Read the model definition and answer for the solid it produces. Units are mm, in the model's axes. Face numbers are marked on the shaded views. A direction names the side the tool comes from. Round coordinates to 2 decimals unless told otherwise and drop trailing zeros. Loops run counter-clockwise (first coordinate to the right, second up) from the corner with the lowest first, then second, coordinate; pieces in that order, holes last. Notation, with made-up numbers: M 47.25,-1 L 80.25,-1 A11 ccw 80.25,7 Z; hole C 60,64.25 d1. An arc over 180 degrees is marked long. Write each question's results on one line, items separated by ' | '.
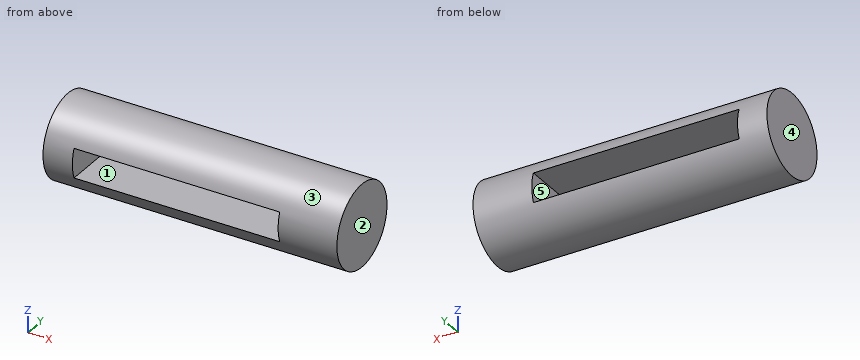
```python
from build123d import *

# Parameters (mm, degrees)
SKETCH1_R           = 7
BOSS_EXTRUDE1_DEPTH = 50
SKETCH2_W           = 35
SKETCH2_H           = 14
CUT_EXTRUDE1_DEPTH  = 2.5


with BuildPart() as part:
    # Sketch1 → Boss-Extrude1 (new body)
    with BuildSketch(Plane(origin=(0, 0, 0), x_dir=(0, 0, -1), z_dir=(1, 0, 0))):
        Circle(SKETCH1_R)
    extrude(amount=BOSS_EXTRUDE1_DEPTH)

    # Sketch2 → Cut-Extrude1 (cut, symmetric)
    with BuildSketch(Plane.XY):
        with Locations((22.5, 0)):
            Rectangle(SKETCH2_W, SKETCH2_H)
    extrude(amount=CUT_EXTRUDE1_DEPTH, both=True, mode=Mode.SUBTRACT)


solid = part.part
```
1. Find section B-B, the plane y = 2.5. Give the vertices of the cut face in (x, z), then the cut area to 3 significant figures.
Completed:
outline: M 0,-6.54 L 50,-6.54 L 50,6.54 L 0,6.54 Z; hole M 5,-2.5 L 40,-2.5 L 40,2.5 L 5,2.5 Z | area: 479 mm2
2. Given P1, Ø8, axis at x = 7, y = 4.5, coming from the +Z side; P2, Ø5, axis at x = 6.5, z = 3.5, coming from the -Y side; P3, Ø1, axis at x = 43.5, y = 5, coming from the +Z side, each flat-ended and moving along its own axis, determine where each tip first touches the part or whether it passes through.
Completed:
P1: stops at z = 6.98 | P2: stops at y = -6.84 | P3: stops at z = 5.36
3. Find section A-A, the plane z = 0. Give the vertices of the cut face in (x, y), then the cut area to 3 significant figures.
Completed:
outline: M 0,-7 L 5,-7 L 5,7 L 0,7 Z; M 40,-7 L 50,-7 L 50,7 L 40,7 Z | area: 210 mm2
4. Find section C-C, the plane x = 33. Give the vertices of the cut face in (y, z).
Completed:
outline: M -6.54,-2.5 A7 ccw 6.54,-2.5 Z; M -6.54,2.5 L 6.54,2.5 A7 ccw Z
5. Determine the mould class of the marked faces 1, 2 and 3 for opening direction Z: released by +Z, released by -Z, zero draft, split by the parting line, or undercut.
Completed:
face 1: undercut | face 2: zero draft | face 3: split by the parting line
6. Which of the six approach directions +Z, -Z, +X, -X, +Y, -Y give full straight-line access (tool end or side, diameter ignored) to the marked faces 4 and 5?
Completed:
face 4: +Z, -Z, -X, +Y, -Y | face 5: +Y, -Y
7. Find the intervals of material crossed by L1, parallel to X at y = 1, z = 0; L2, parallel to Z at x = 36, y = 5.25; L3, parallel to Z at x = 12, y = -2.75, in increasing order.
Completed:
L1: x = 0 to 5, 40 to 50 | L2: z = -4.63 to -2.5, 2.5 to 4.63 | L3: z = -6.44 to -2.5, 2.5 to 6.44
8. Find section D-D, the plane y = 0. Give the vertices of the cut face in (x, z).
Completed:
outline: M 0,-7 L 50,-7 L 50,7 L 0,7 Z; hole M 5,-2.5 L 40,-2.5 L 40,2.5 L 5,2.5 Z
